Geometry check sheet. Reference: the model listing, model coordinates, mm. A direction names the side the tool comes from. Give positions to 0.01 mm unless a question says otherwise; leave off trailing zeros. Write each loop counter-clockwise with the first axis right and the second up, starting at its lowest first coordinate (ties: lowest second). Pieces come first, ordered by that corner, then holes. Notation, with made-up numbers: (72.5, -13.5) - (93.5, -13.5) arc R24 ccw to (93.5, 0.5) - close; hole circle Ø3 at (69.25, -16). An arc over 180 degrees is marked (long way). Write item = value, one per line. Start each with the question number.
(1) Section check A-A, the plane z = 8.5. Enter the section's corners in (x, y).
(2) Draft check along Y on faces 4 (the flat face through (10, 0, 29)), 5 (the flat face through (10, -64, 58)), 6 (the flat face through (10, -120, 68)). Enter one of: pulls with the +Y half, pulls with the -Y half, needs draft (parallel to the pull), parting line crosses it, or undercut.
(3) Access from +Z, -Z, +X, -X, +Y, -Y to the whole of each face (thin tool, end or side, straight path). Record for faces 1 (the flat face through (20, -66, 29)), 2 (the cylindrical face through (14.292, -8.648, 62.93)), 3 (the flat face through (10, -57, 10)).
(4) Section check C-C, the plane y = -65. Enter the section's corners in (x, z).
(5) Section check B-B, the plane x = 10. Enter the section's corners in (y, z).
(6) Section check D-D, the plane z = 25. Enter the section's corners in (x, y) (3 decimals).
(7) Depth check by flat-ended pin: pin 1 Ø1 at (x, y) = (4, -50) entering from +Z; pin 2 Ø4 at (y, z) = (-30.5, 60.5) entering from +X. Enter the tip coordinate at first touch or a pass-through.
(8) Thickness scan on L1, parallel to Y at x = 15.75, z = 9; L2, parallel to Z at x = 8, y = -15; L3, parallel to Y at x = 7.5, z = 22. Record the ranges inside material, lowest first.
```python
from build123d import *

# Parameters (mm, degrees)
F0_W     = 20
F0_H     = 130
F1_DEPTH = 58
F3_DEPTH = 20.001
F4_R     = 4.5
F5_DEPTH = 10


with BuildPart() as f1:
    # F0 (on Top) → F1 (new body)
    with BuildSketch(Plane.XY):
        with Locations((10, -65)):
            Rectangle(F0_W, F0_H)
    extrude(amount=F1_DEPTH)

    # F2 (on face) → F3 (cut, through all)
    with BuildSketch(Plane.YZ.offset(20)):
        with BuildLine():
            Line((-57, 0), (-57, 20))
            ThreePointArc((-57, 20), (-65, 28), (-73, 20))
            Line((-73, 20), (-73, 0))
            Line((-73, 0), (-57, 0))
        make_face()
    extrude(amount=-F3_DEPTH, mode=Mode.SUBTRACT)

    # F4 (on face) → F5 (join)
    with BuildSketch(Plane.XY.offset(58)):
        with Locations((10, -10)):
            Circle(F4_R)
        with Locations((10, -120)):
            Circle(F4_R)
    extrude(amount=F5_DEPTH)


solid = f1.part
```
Model answer:
q1.outline = (0, -130) - (20, -130) - (20, -73) - (0, -73) - close; (0, -57) - (20, -57) - (20, 0) - (0, 0) - close
q2.face_4 = pulls with the +Y half
q2.face_5 = undercut
q2.face_6 = needs draft
q3.face_1 = +Z, -Z, +X, +Y, -Y
q3.face_2 = +Z
q3.face_3 = -Z, +X, -X
q4.outline = (0, 28) - (20, 28) - (20, 58) - (0, 58) - close
q5.outline = (-130, 0) - (-73, 0) - (-73, 20) arc R8 cw to (-57, 20) - (-57, 0) - (0, 0) - (0, 58) - (-5.5, 58) - (-5.5, 68) - (-14.5, 68) - (-14.5, 58) - (-115.5, 58) - (-115.5, 68) - (-124.5, 68) - (-124.5, 58) - (-130, 58) - close
q6.outline = (0, -130) - (20, -130) - (20, -71.245) - (0, -71.245) - close; (0, -58.755) - (20, -58.755) - (20, 0) - (0, 0) - close
q7.pin_1 = 58
q7.pin_2 = through
q8.L1 = -130 to -73, -57 to 0
q8.L2 = 0 to 58
q8.L3 = -130 to -72.75, -57.25 to 0
